CAD build for the part. Positions are in the model's coordinates, mm. Face numbers are marked on the shaded views. A direction names the side the tool comes from. Give positions to 0.01 mm unless a question says otherwise; leave off trailing zeros. Write each loop counter-clockwise with the first axis right and the second up, starting at its lowest first coordinate (ties: lowest second). Pieces come first, ordered by that corner, then holes. Notation, with made-up numbers: (42, 5.25) - (80, 5.25) arc R18 cw to (80, 32.25) - close; hole circle Ø4 at (-18, 30.25). An arc over 180 degrees is marked (long way). Put each result on its own line as item: value. Start each with the question number.
1. Tool access for the marked faces 1 and 2: list every direction of +Z, -Z, +X, -X, +Y, -Y with a clear straight run to the whole face (end or side of a thin tool).
2. Cut at A-A on z = 5. List the corners of the cut face in (x, y).
3. Wall check: line 1 (Y direction, x = -0.5, z = 23.5); line 2 (X direction, y = -1.5, z = 8); line 3 (Y direction, x = 8, z = 12). Give the ranges that are in metal, low to high.
4. Drop flat-ended pins along their axis: pin 1 (11 mm diameter, centred on x = 2.5, y = 2.5, fed in from +Z); pin 2 (2 mm diameter, centred on y = 3, z = 24.5, fed in from +X); pin 3 (2 mm diameter, centred on y = -8, z = 6, fed in from +X). Give the stop position or say it passes through.
5. Cut at D-D on y = 6. List the corners of the cut face in (x, z), and give its area (3 significant figures).
6. Cut at C-C on x = 4. List the corners of the cut face in (y, z), and give its area (3 significant figures).
7. Cut at B-B on z = 15.5. List the corners of the cut face in (x, y), and give its area (3 significant figures).
from build123d import *

# Parameters (mm, degrees)
F1_DEPTH = 30.4
F2_DEPTH = 2
F3_W     = 6.9
F3_H     = 6.9
F4_DEPTH = 50
F5_R     = 1
F6_DEPTH = 30.4


# Not quite as in the source:
# - a feature names something its author has since deleted; it is built from what else it names


with BuildPart() as f1:
    # F0 (on Top) → F1 (new body)
    with BuildSketch(Plane.XY):
        with BuildLine():
            ThreePointArc((0, -18), (-18, 0), (0, 18))
            Line((0, 18), (-27.8, 18))
            Line((-27.8, 18), (-27.8, -18))
            Line((-27.8, -18), (0, -18))
        make_face()
        with BuildLine():
            ThreePointArc((0, -17.25), (-17.25, 0), (0, 17.25))
            Line((0, 17.25), (0, 18))
            ThreePointArc((0, 18), (-18, 0), (0, -18))
            Line((0, -18), (0, -17.25))
        make_face()
        with BuildLine():
            ThreePointArc((0, 17.25), (12.1975919755, 12.1975919755), (17.25, 0))
            ThreePointArc((17.25, 0), (12.1975919755, -12.1975919755), (0, -17.25))
            Line((0, -17.25), (0, -18))
            ThreePointArc((0, -18), (12.7279220614, -12.7279220614), (18, 0))
            ThreePointArc((18, 0), (12.7279220614, 12.7279220614), (0, 18))
            Line((0, 18), (0, 17.25))
        make_face()
    extrude(amount=F1_DEPTH)

    # F0 (on Top) → F2 (join)
    with BuildSketch(Plane.XY):
        with BuildLine():
            ThreePointArc((0, -17.25), (12.1975919755, -12.1975919755), (17.25, 0))
            ThreePointArc((17.25, 0), (12.1975919755, 12.1975919755), (0, 17.25))
            Line((0, 17.25), (0, 12.2))
            ThreePointArc((0, 12.2), (8.6267027305, 8.6267027305), (12.2, 0))
            ThreePointArc((12.2, 0), (8.6267027305, -8.6267027305), (0, -12.2))
            Line((0, -12.2), (0, -17.25))
        make_face()
        with BuildLine():
            Line((0, 12.2), (0, 17.25))
            ThreePointArc((0, 17.25), (-17.25, 0), (0, -17.25))
            Line((0, -17.25), (0, -12.2))
            ThreePointArc((0, -12.2), (-12.2, 0), (0, 12.2))
        make_face()
    extrude(amount=F2_DEPTH)

    # F3 (on face) → F4 (cut)
    with BuildSketch(Plane.XZ.offset(18)):
        with Locations((-22.45, 25.05)):
            Rectangle(F3_W, F3_H)
        with Locations((-22.45, 5.35)):
            Rectangle(F3_W, F3_H)
    extrude(amount=-F4_DEPTH, mode=Mode.SUBTRACT)

    # F5
    f5_edges = [f1.edges().sort_by_distance(p)[0] for p in [
        (-27.8, 18, 15.2),
        (-27.8, -18, 15.2),
    ]]
    fillet(f5_edges, radius=F5_R)



with BuildPart() as f2:
    # F0 (on Top) → F2, piece 2 (new body)
    with BuildSketch(Plane.XY):
        with BuildLine():
            ThreePointArc((11.2, 0), (7.9195959493, 7.9195959493), (0, 11.2))
            Line((0, 11.2), (0, 5))
            ThreePointArc((0, 5), (3.5355339059, 3.5355339059), (5, 0))
            ThreePointArc((5, 0), (3.5355339059, -3.5355339059), (0, -5))
            Line((0, -5), (0, -11.2))
            ThreePointArc((0, -11.2), (7.9195959493, -7.9195959493), (11.2, 0))
        make_face()
        with BuildLine():
            Line((0, 5), (0, 11.2))
            ThreePointArc((0, 11.2), (-11.2, 0), (0, -11.2))
            Line((0, -11.2), (0, -5))
            ThreePointArc((0, -5), (-5, 0), (0, 5))
        make_face()
    extrude(amount=F2_DEPTH)


with BuildPart() as f1_1:
    add(f1.part)

    add(f2.part)  # F6 merges F2
    # F0 (on Top) → F6 (join, through all)
    with BuildSketch(Plane.XY):
        with BuildLine():
            ThreePointArc((12.2, 0), (8.6267027305, 8.6267027305), (0, 12.2))
            Line((0, 12.2), (0, 11.2))
            ThreePointArc((0, 11.2), (7.9195959493, 7.9195959493), (11.2, 0))
            ThreePointArc((11.2, 0), (7.9195959493, -7.9195959493), (0, -11.2))
            Line((0, -11.2), (0, -12.2))
            ThreePointArc((0, -12.2), (8.6267027305, -8.6267027305), (12.2, 0))
        make_face()
        with BuildLine():
            Line((0, 11.2), (0, 12.2))
            ThreePointArc((0, 12.2), (-12.2, 0), (0, -12.2))
            Line((0, -12.2), (0, -11.2))
            ThreePointArc((0, -11.2), (-11.2, 0), (0, 11.2))
        make_face()
    extrude(amount=F6_DEPTH)


solid = f1_1.part
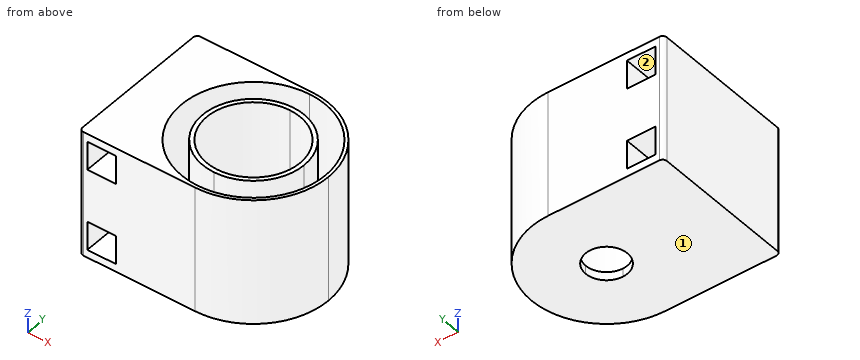
Report:
1. face 1: -Z, +X, -X, +Y, -Y
1. face 2: +Y, -Y
2. outline: (-27.8, -17) arc R1 ccw to (-26.8, -18) - (-25.9, -18) - (-25.9, 18) - (-26.8, 18) arc R1 ccw to (-27.8, 17) - close; (-19, -18) - (0, -18) arc R18 ccw to (0, 18) - (-19, 18) - close; circle Ø24.4 at (0, 0); hole circle Ø34.5 at (0, 0); hole circle Ø22.4 at (0, 0)
3. line 1: y = -18 to -17.24, -12.19 to -11.19, 11.19 to 12.19, 17.24 to 18
3. line 2: x = -27.8 to -25.9, -19 to -17.18, -12.11 to -11.1, 11.1 to 12.11, 17.18 to 17.94
3. line 3: y = -16.12 to -15.28, -9.21 to -7.84, 7.84 to 9.21, 15.28 to 16.12
4. pin 1: stops at z = 2
4. pin 2: stops at x = 17.89
4. pin 3: stops at x = 16.58
5. outline: (-27.8, 0) - (16.97, 0) - (16.97, 30.4) - (16.17, 30.4) - (16.17, 2) - (10.62, 2) - (10.62, 30.4) - (9.46, 30.4) - (9.46, 2) - (-9.46, 2) - (-9.46, 30.4) - (-10.62, 30.4) - (-10.62, 2) - (-16.17, 2) - (-16.17, 30.4) - (-27.8, 30.4) - close; hole (-25.9, 1.9) - (-19, 1.9) - (-19, 8.8) - (-25.9, 8.8) - close; hole (-25.9, 21.6) - (-19, 21.6) - (-19, 28.5) - (-25.9, 28.5) - close
5. area: 413 mm²
6. outline: (-17.55, 0) - (-3, 0) - (-3, 2) - (-10.46, 2) - (-10.46, 30.4) - (-11.53, 30.4) - (-11.53, 2) - (-16.78, 2) - (-16.78, 30.4) - (-17.55, 30.4) - close; (3, 0) - (17.55, 0) - (17.55, 30.4) - (16.78, 30.4) - (16.78, 2) - (11.53, 2) - (11.53, 30.4) - (10.46, 30.4) - (10.46, 2) - (3, 2) - close
6. area: 162 mm²
7. outline: (-27.8, -17) arc R1 ccw to (-26.8, -18) - (0, -18) arc R18 ccw to (0, 18) - (-26.8, 18) arc R1 ccw to (-27.8, 17) - close; circle Ø24.4 at (0, 0); hole circle Ø34.5 at (0, 0); hole circle Ø22.4 at (0, 0)
7. area: 648 mm²
